```python
from build123d import *

# Parameters (mm, degrees)
F1_W              = 40.6
F1_H              = 19.8
F2_DEPTH          = 36.6
F3_R              = 7
F4_DEPTH          = 2.5
F5_R              = 4
F6_DEPTH          = 2.5
F7_R              = 12
F8_DEPTH          = 2
F10_W             = 6.4
F10_H             = 19.8
F11_DEPTH         = 2
F13_DEPTH         = 4
F13_COPIES2_COUNT = 2
F14_R             = 1
F16_DEPTH         = 0.5


# Not quite as in the source:
# - a pattern or mirror of a feature is missing from the dataset's text; its kind, count and spacing are read off the source's solid


with BuildPart() as f2:
    # F1 (on Top) → F2 (new body)
    with BuildSketch(Plane.XY):
        Rectangle(F1_W, F1_H)
    extrude(amount=F2_DEPTH)

    # F3 (on face) → F4 (join)
    with BuildSketch(Plane.XY.offset(36.6)):
        with Locations((10.64, 0)):
            Circle(F3_R)
    extrude(amount=F4_DEPTH)

    # F5 (on face) → F6 (join)
    with BuildSketch(Plane.XY.offset(39.1)):
        with Locations((10.64, 0)):
            Circle(F5_R)
    extrude(amount=F6_DEPTH)

    # F7 (on face) → F8 (join)
    with BuildSketch(Plane.XY.offset(41.6)):
        with Locations((10.64, 0)):
            Circle(F7_R)
    extrude(amount=F8_DEPTH)

    # F10 (on offset) → F11 (join)
    with BuildSketch(Plane.XY.offset(26.8)):
        with Locations((23.5, 0)):
            Rectangle(F10_W, F10_H)
    f11 = extrude(amount=F11_DEPTH)

    # F11_copies: F11 across plane
    add(f11.mirror(Plane(origin=(0, 0, 0), x_dir=(0, 0, -1), z_dir=(-1, 0, 0))))

    # F12 (on offset) → F13 (cut)
    with BuildSketch(Plane.XY.offset(26.8)):
        with BuildLine():
            Line((26.7, -3.5), (25.7956503376, -3.5))
            ThreePointArc((25.7956503376, -3.5), (22.01, -5), (25.7956503376, -6.5))
            Line((25.7956503376, -6.5), (26.7, -6.5))
            Line((26.7, -6.5), (26.7, -3.5))
        make_face()
    f13 = extrude(amount=F13_DEPTH, mode=Mode.SUBTRACT)

    # F13_copies: F13 across plane
    add(f13.mirror(Plane(origin=(0, 0, 0), x_dir=(0, 0, -1), z_dir=(-1, 0, 0))), mode=Mode.SUBTRACT)

    # F13_copies1: F13 across plane
    add(f13.mirror(Plane.ZX), mode=Mode.SUBTRACT)

    # F13_copies2: F13 ×2 about axis
    f13_copies2_axis = Axis((0, 0, 0), (0, 0, 1))
    for i in range(1, F13_COPIES2_COUNT):
        add(f13.rotate(f13_copies2_axis, i * 360 / F13_COPIES2_COUNT), mode=Mode.SUBTRACT)

    # F14
    f14_edges = [f2.edges().sort_by_distance(p)[0] for p in [
        (-20.3, -9.9, 13.4),
        (0, -9.9, 0),
        (-20.3, 0, 0),
        (-20.3, 9.9, 13.4),
        (0, 9.9, 0),
        (20.3, 0, 0),
        (20.3, 9.9, 13.4),
        (20.3, -9.9, 13.4),
        (-20.3, 0, 36.6),
        (0, 9.9, 36.6),
        (0, -9.9, 36.6),
        (20.3, -9.9, 32.7),
        (20.3, 0, 36.6),
        (20.3, 9.9, 32.7),
        (26.7, -9.9, 27.8),
        (26.7, 9.9, 27.8),
        (-20.3, 9.9, 32.7),
        (-26.7, 9.9, 27.8),
        (-20.3, -9.9, 32.7),
        (-26.7, -9.9, 27.8),
    ]]
    fillet(f14_edges, radius=F14_R)

    # F15 (on Front) → F16 (join, symmetric)
    with BuildSketch(Plane.XZ):
        Polygon((26.7, 28.8), (25.8339745962, 30.3), (20.3, 30.3), (20.3, 28.8), align=None)
    f16 = extrude(amount=F16_DEPTH, both=True)

    # F16_copies: F16 across plane
    add(f16.mirror(Plane(origin=(0, 0, 0), x_dir=(0, 0, -1), z_dir=(-1, 0, 0))))


solid = f2.part
```
Verification items for the finished model (mm, model axes). A direction names the side the tool comes from. Coordinates: 2 decimals unless noted, no trailing zeros. Loops run counter-clockwise (first coordinate to the right, second up) from the corner with the lowest first, then second, coordinate; pieces in that order, holes last. Notation, with made-up numbers: (-29.75, 36.25) -> (-2.75, 36.25) arc R10 cw to (-2.75, 52.25) -> close; hole circle Ø4 at (50.5, -25.75). An arc over 180 degrees is marked (long way). Answer in a Markdown table with one row per item.
1) Scan lines: line 1 along Y through (x, z) = (24, 28); line 2 along Z through (x, y) = (1, -1.5); line 3 along Z through (x, y) = (15, -4.75). Record each from-to range of solid material in increasing order. Write a range as from..to.
The answers:
| item | result |
|---|---|
| line 1 | y = -9.9..-7.18, -2.82..2.82, 7.18..9.9 |
| line 2 | z = 0..36.6, 41.6..43.6 |
| line 3 | z = 0..39.1, 41.6..43.6 |
2) Depth check by flat-ended pin: P1, Ø1, axis at x = -26.5, z = 28.5, coming from the +Y side; P2, Ø0.8, axis at x = -24, y = 0, coming from the +Z side; P3, Ø1, axis at x = -26, z = 28, coming from the -Y side. Enter the tip coordinate at first touch or a pass-through.
The answers:
| item | result |
|---|---|
| P1 | stops at y = 9.85 |
| P2 | stops at z = 30.3 |
| P3 | stops at y = -9.9 |
3) Section check C-C (z = 3.5). Record the cut outline in (x, y).
The answers:
| item | result |
|---|---|
| outline | (-20.3, -8.9) arc R1 ccw to (-19.3, -9.9) -> (19.3, -9.9) arc R1 ccw to (20.3, -8.9) -> (20.3, 8.9) arc R1 ccw to (19.3, 9.9) -> (-19.3, 9.9) arc R1 ccw to (-20.3, 8.9) -> close |
4) Draft check along Z on faces 4 (the face through (22, -6, 28.8)), 5 (the face through (-5, 0, 36.6)), 6 (the face through (-22, 6, 28.8)), 7 (the face through (-23, 0.5, 30)). Enter one of: released by +Z, released by -Z, zero draft, split by the parting line, or undercut.
The answers:
| item | result |
|---|---|
| face 4 | undercut |
| face 5 | undercut |
| face 6 | released by +Z |
| face 7 | zero draft |
5) Section check D-D (x = 10.64). Record the cut outline in (y, z).
The answers:
| item | result |
|---|---|
| outline | (-12, 41.6) -> (-4, 41.6) -> (-4, 39.1) -> (-7, 39.1) -> (-7, 36.6) -> (-8.9, 36.6) arc R1 ccw to (-9.9, 35.6) -> (-9.9, 1) arc R1 ccw to (-8.9, 0) -> (8.9, 0) arc R1 ccw to (9.9, 1) -> (9.9, 35.6) arc R1 ccw to (8.9, 36.6) -> (7, 36.6) -> (7, 39.1) -> (4, 39.1) -> (4, 41.6) -> (12, 41.6) -> (12, 43.6) -> (-12, 43.6) -> close |
6) Section check B-B (y = -5). Record the cut outline in (x, z), and give its area (3 significant figures).
The answers:
| item | result |
|---|---|
| outline | (-22.01, 26.8) -> (-20.3, 26.8) -> (-20.3, 1) arc R1 ccw to (-19.3, 0) -> (19.3, 0) arc R1 ccw to (20.3, 1) -> (20.3, 26.8) -> (22.01, 26.8) -> (22.01, 28.8) -> (20.3, 28.8) -> (20.3, 35.6) arc R1 ccw to (19.3, 36.6) -> (15.54, 36.6) -> (15.54, 39.1) -> (5.74, 39.1) -> (5.74, 36.6) -> (-19.3, 36.6) arc R1 ccw to (-20.3, 35.6) -> (-20.3, 28.8) -> (-22.01, 28.8) -> close; (-0.27, 41.6) -> (21.55, 41.6) -> (21.55, 43.6) -> (-0.27, 43.6) -> close |
| area | 1,560 mm2 |
7) Access from +Z, -Z, +X, -X, +Y, -Y to the whole of each face (thin tool, end or side, straight path). Record for faces 1 (the face through (14, -3, 39.1)), 2 (the face through (0, -9.9, 18)), 3 (the face through (23, -0.5, 30)).
The answers:
| item | result |
|---|---|
| face 1 | none |
| face 2 | -Z, +X, -X, -Y |
| face 3 | +X, -Y |
8) Section check A-A (x = -24.2). Record the cut outline in (y, z).
The answers:
| item | result |
|---|---|
| outline | (-9.9, 26.8) -> (-7.19, 26.8) -> (-7.19, 28.8) -> (-9.9, 28.8) -> close; (-2.81, 26.8) -> (2.81, 26.8) -> (2.81, 28.8) -> (0.5, 28.8) -> (0.5, 30.3) -> (-0.5, 30.3) -> (-0.5, 28.8) -> (-2.81, 28.8) -> close; (7.19, 26.8) -> (9.9, 26.8) -> (9.9, 28.8) -> (7.19, 28.8) -> close |
